from build123d import *

# Parameters (mm, degrees)
SKETCH1_R           = 1.0922
SKETCH1_R_2         = 2.1
BOSS_EXTRUDE1_DEPTH = 3.175


with BuildPart() as part:
    # Sketch1 → Boss-Extrude1 (new body)
    with BuildSketch(Plane(origin=(0, 0, 0), x_dir=(1, 0, 0), z_dir=(0, 1, 0))):
        with BuildLine():
            Line((0, 39.37), (266.7, 39.37))
            ThreePointArc((266.7, 39.37), (306.07, 0), (266.7, -39.37))
            Line((266.7, -39.37), (0, -39.37))
            ThreePointArc((0, -39.37), (-39.37, 0), (0, 39.37))
        make_face()
        with Locations((38.1, 36.195)):
            Circle(SKETCH1_R, mode=Mode.SUBTRACT)
        with Locations((228.6, 36.195)):
            Circle(SKETCH1_R, mode=Mode.SUBTRACT)
        with Locations((38.1, -36.195)):
            Circle(SKETCH1_R, mode=Mode.SUBTRACT)
        with Locations((228.6, -36.195)):
            Circle(SKETCH1_R, mode=Mode.SUBTRACT)
        with Locations((-36.195, 0)):
            Circle(SKETCH1_R, mode=Mode.SUBTRACT)
        with Locations((304.4825, 0)):
            Circle(SKETCH1_R, mode=Mode.SUBTRACT)
        with Locations((266.7, 0)):
            Circle(SKETCH1_R_2, mode=Mode.SUBTRACT)
        with Locations((0, -6.35)):
            Circle(SKETCH1_R_2, mode=Mode.SUBTRACT)
        with Locations((0, 6.35)):
            Circle(SKETCH1_R_2, mode=Mode.SUBTRACT)
    extrude(amount=BOSS_EXTRUDE1_DEPTH)


solid = part.part
Build history of the part. All positions in model axes, mm. Give positions to 0.01 mm unless a question says otherwise; leave off trailing zeros. Order: outer loops, then holes, each group sorted by start corner. A loop starts at its lowest first (then second) coordinate and runs counter-clockwise, first axis right, second up. Notation, with made-up numbers: M -11.75,69.5 L 17.25,69.5 A20 cw 17.25,104.5 Z; hole C 56,-34.75 d9. An arc over 180 degrees is marked long. Use one line per item in the form item = value.
1) Saw through at B-B (z = -14.5). Give the cut face in (x, y) (3 decimals), plus the area to 3 significant figures.
Calculated:
outline = M -36.603,0 L 303.303,0 L 303.303,3.175 L -36.603,3.175 Z
area = 1,080 mm2
2) Probe probe 1 along Z at (x, y) = (38.1, 2); probe 2 along X at (y, z) = (2, 0); probe 3 along Z at (x, y) = (268.5, 0.4). List the from-to ranges inside material, lowest first.
Calculated:
probe_1 = -39.37 to -37.29, -35.1 to 35.1, 37.29 to 39.37
probe_2 = -39.37 to -37.29, -35.1 to 264.6, 268.8 to 303.39, 305.57 to 306.07
probe_3 = -39.33 to -1.08, 1.08 to 39.33
3) Saw through at C-C (x = -7). Give the cut face in (y, z) (3 decimals), plus the area to 3 significant figures.
Calculated:
outline = M 0,-38.743 L 3.175,-38.743 L 3.175,38.743 L 0,38.743 Z
area = 246 mm2
4) Saw through at A-A (y = 2.2). State how many separate pieces and enclosed holes the cut face has, plus the area to 3 significant figures.
Calculated:
separate_pieces = 1
enclosed_holes = 9
area = 25,800 mm2
5) Drop flat-ended pins along their axis: pin 1 (1.7 mm diameter, centred on x = 304.48, z = 0, fed in from -Y); pin 2 (5.5 mm diameter, centred on x = 0, z = 6.35, fed in from -Y); pin 3 (1 mm diameter, centred on y = 2.5, z = -28.5, fed in from -X); pin 4 (1.5 mm diameter, centred on y = 0.5, z = 30.5, fed in from +X). Give the stop position or say it passes through.
Calculated:
pin_1 = through
pin_2 = 0
pin_3 = -27.68
pin_4 = 292.49
